Geometry: final body of the model. Coordinates: model frame, mm. Give positions to 0.01 mm unless a question says otherwise; leave off trailing zeros. Write each loop counter-clockwise with the first axis right and the second up, starting at its lowest first coordinate (ties: lowest second). Pieces come first, ordered by that corner, then holes. Notation, with made-up numbers: (77.5, 39) - (96.5, 39) arc R13 cw to (96.5, 49) - close; hole circle Ø2 at (87.25, -19). An arc over 180 degrees is marked (long way). Return JSON: item names as keys, results as strings.
from build123d import *

# Parameters (mm, degrees)
SKETCH_1_R          = 55
EXTRUDE_1_DEPTH     = 2
SKETCH_2_R          = 1.65
CUT_EXTRUDE_1_DEPTH = 14
SKETCH_3_R          = 42.5
CUT_EXTRUDE_2_DEPTH = 14


with BuildPart() as part:
    # 草图1 → 凸台-拉伸1 (new body)
    with BuildSketch(Plane(origin=(0, 0, 0), x_dir=(1, 0, 0), z_dir=(0, 1, 0))):
        Circle(SKETCH_1_R)
    extrude(amount=EXTRUDE_1_DEPTH)

    # 草图2 → 切除-拉伸1 (cut)
    with BuildSketch(Plane(origin=(0, 2, 0), x_dir=(1, 0, 0), z_dir=(0, 1, 0))):
        with Locations((-48.898985831, -5.869555746)):
            Circle(SKETCH_2_R)
        with Locations((-5.869555746, 48.898985831)):
            Circle(SKETCH_2_R)
        with Locations((48.898985831, 5.869555746)):
            Circle(SKETCH_2_R)
        with Locations((5.869555746, -48.898985831)):
            Circle(SKETCH_2_R)
    extrude(amount=-CUT_EXTRUDE_1_DEPTH, mode=Mode.SUBTRACT)

    # 草图3 → 切除-拉伸2 (cut)
    with BuildSketch(Plane(origin=(0, 2, 0), x_dir=(1, 0, 0), z_dir=(0, 1, 0))):
        Circle(SKETCH_3_R)
    extrude(amount=-CUT_EXTRUDE_2_DEPTH, mode=Mode.SUBTRACT)


solid = part.part
Q1. Section query C-C, the plane y = 1.15. Return the cut outline in (x, z).
Answer key:
{"outline": "circle Ø110 at (0, 0); hole circle Ø3.3 at (-48.9, 5.87); hole circle Ø85 at (0, 0); hole circle Ø3.3 at (-5.87, -48.9); hole circle Ø3.3 at (5.87, 48.9); hole circle Ø3.3 at (48.9, -5.87)"}
Q2. Mould query, pull axis X, two halves, no side actions, for faces 1 (the cylindrical face through (47.25, 1.01, -5.94)), 2 (the flat face through (-41, 2, 12)), 3 (the cylindrical face through (-11.923, 0.986, 53.692)), 4 (the cylindrical face through (-7.1, 1, -50)). Classes: pulls with the +X half, pulls with the -X half, needs draft (parallel to the pull), parting line crosses it, or undercut.
Answer key:
{"face 1": "undercut", "face 2": "needs draft", "face 3": "parting line crosses it", "face 4": "undercut"}
Q3. Material intervals for probe 1 along Z at (x, y) = (-0.5, 1.6); probe 2 along X at (y, z) = (0.9, -48); probe 3 along Z at (x, y) = (-22.5, 0.1), sorted ascending. Write a range as [from, to].
Answer key:
{"probe 1": "z = [-55, -42.5], [42.5, 55]", "probe 2": "x = [-26.85, -7.25], [-4.49, 26.85]", "probe 3": "z = [-50.19, -36.06], [36.06, 50.19]"}
Q4. Section query A-A, the plane z = 0. Return the cut outline in (x, y).
Answer key:
{"outline": "(-55, 0) - (-42.5, 0) - (-42.5, 2) - (-55, 2) - close; (42.5, 0) - (55, 0) - (55, 2) - (42.5, 2) - close"}
Q5. Section query B-B, the plane x = 0. Return the cut outline in (y, z), plus the area to 3 significant figures.
Answer key:
{"outline": "(0, -55) - (2, -55) - (2, -42.5) - (0, -42.5) - close; (0, 42.5) - (2, 42.5) - (2, 55) - (0, 55) - close", "area": "50.0 mm^2"}
Q6. Section query D-D, the plane z = 46. Return the cut outline in (x, y).
Answer key:
{"outline": "(-30.15, 0) - (30.15, 0) - (30.15, 2) - (-30.15, 2) - close"}
Q7. Pin query (flat end, axial travel): P1, Ø5, axis at x = 42.5, z = 40, coming from the +Y side; P2, Ø1, axis at x = 21.5, y = 1, coming from the -Z side. Return the tip coordinate at first contact, or that it passes through.
Answer key:
{"P1": "passes through", "P2": "stops at z = -50.83"}
